```python
from build123d import *

# Parameters (mm, degrees)
F1_DEPTH = 63.5
F0_R     = 63.6308259599
F0_R_2   = 52.2581940634
F0_W     = 24.2178440094
F0_H     = 175.5797639489
F0_W_2   = 299.6964156628
F0_H_2   = 33.2996025681
F2_DEPTH = 6.35
F5_DEPTH = 25.4
F6_DEPTH = 19.05


# Not quite as in the source:
# - the program builds the solid bodies; features that only make, move or delete a surface that nothing else refers to are left out


with BuildPart() as f1:
    # F0 (on Front) → F1 (new body)
    with BuildSketch(Plane.XZ):
        Polygon((-969.1663980484, 198.6485360199), (-921.1349980484, 198.6485360199), (907.6650019516, 198.6485360199), (955.6964019516, 198.6485360199), (956.6172361374, 198.6485360199), (956.6172361374, 246.6799360199), (-969.1663980484, 246.6799360199), align=None)
        Polygon((-921.1349980484, -371.5092837811), (-921.1349980484, 198.6485360199), (-969.1663980484, 198.6485360199), (-969.1663980484, -410.9517233025), (-921.1349980484, -410.9517233025), (-921.1349980484, -410.9514639801), align=None)
        Polygon((-921.1349980484, -410.9517233025), (-969.1663980484, -410.9517233025), (-969.1663980484, -458.9831233025), (955.726981163, -458.9831233025), (955.726981163, -410.9517233025), (955.6964019516, -410.9517233025), (907.6650019516, -410.9517233025), align=None)
        Polygon((955.6964019516, 198.6485360199), (907.6650019516, 198.6485360199), (907.6650019516, -410.9514639801), (907.6650019516, -410.9517233025), (955.6964019516, -410.9517233025), align=None)
    extrude(amount=F1_DEPTH)

    # F0 (on Front) → F2 (join)
    with BuildSketch(Plane.XZ):
        Polygon((907.6650019516, 198.6485360199), (-921.1349980484, 198.6485360199), (-921.1349980484, -371.5092837811), (-921.1349980484, -410.9514639801), (-31.4717553556, -410.9514639801), (907.6650019516, -410.9514639801), align=None)
        Polygon((-789.5849161051, -398.2566583191), (-795.2640652657, -368.8750267029), (-420.4561412334, -296.4287400246), (-420.4561412334, -326.9080892764), align=None, mode=Mode.SUBTRACT)
        Polygon((210.169616585, -380.4944990589), (206.6856175661, -339.3833041191), (563.899576664, -309.1109395027), (566.059074651, -350.3343802749), align=None, mode=Mode.SUBTRACT)
        Polygon((235.5920225382, -246.5991973877), (81.9196328521, -266.643434763), (78.3429656397, -239.222336751), (239.8227507102, -218.1597428141), align=None, mode=Mode.SUBTRACT)
        with Locations((470.1542854309, -190.9026801586)):
            Circle(F0_R, mode=Mode.SUBTRACT)
        with Locations((836.3508582115, -221.3210761547)):
            Circle(F0_R_2, mode=Mode.SUBTRACT)
        with Locations((-737.8122806549, 54.1574768722)):
            Rectangle(F0_W, F0_H, mode=Mode.SUBTRACT)
        Polygon((-614.0667200089, 62.5602602959), (-606.2821745872, 91.4887040854), (-299.1916835308, 14.3223749474), (-307.1056894279, -17.1721380653), align=None, mode=Mode.SUBTRACT)
        Polygon((777.5867510857, 41.2790888272), (818.6616301537, 58.8090009987), (872.9156851768, -56.7944645882), (832.5127084301, -75.7560529142), align=None, mode=Mode.SUBTRACT)
        Polygon((-132.3649287224, 135.8928531408), (109.8140254617, 135.8928531408), (167.3315316439, 81.402592361), (-68.7929466367, 81.402592361), align=None, mode=Mode.SUBTRACT)
        with Locations((625.9579211473, 125.2975575626)):
            Rectangle(F0_W_2, F0_H_2, mode=Mode.SUBTRACT)
        Polygon((907.6650019516, -410.9517233025), (907.6650019516, -410.9514639801), (-31.4717553556, -410.9514639801), (-921.1349980484, -410.9514639801), (-921.1349980484, -410.9517233025), align=None)
    extrude(amount=F2_DEPTH)

    # F0 (on Front) → F5 (join)
    with BuildSketch(Plane.XZ):
        with Locations((625.9579211473, 125.2975575626)):
            Rectangle(F0_W_2, F0_H_2)
        Polygon((167.3315316439, 81.402592361), (109.8140254617, 135.8928531408), (-132.3649287224, 135.8928531408), (-68.7929466367, 81.402592361), align=None)
        Polygon((-299.1916835308, 14.3223749474), (-606.2821745872, 91.4887040854), (-614.0667200089, 62.5602602959), (-307.1056894279, -17.1721380653), align=None)
        Polygon((-420.4561412334, -296.4287400246), (-795.2640652657, -368.8750267029), (-789.5849161051, -398.2566583191), (-420.4561412334, -326.9080892764), align=None)
        Polygon((78.3429656397, -239.222336751), (81.9196328521, -266.643434763), (235.5920225382, -246.5991973877), (239.8227507102, -218.1597428141), align=None)
        Polygon((563.899576664, -309.1109395027), (206.6856175661, -339.3833041191), (210.169616585, -380.4944990589), (566.059074651, -350.3343802749), align=None)
        with Locations((-737.8122806549, 54.1574768722)):
            Rectangle(F0_W, F0_H)
        Polygon((872.9156851768, -56.7944645882), (818.6616301537, 58.8090009987), (777.5867510857, 41.2790888272), (832.5127084301, -75.7560529142), align=None)
    extrude(amount=F5_DEPTH)

    # F0 (on Front) → F6 (join)
    with BuildSketch(Plane.XZ):
        with Locations((470.1542854309, -190.9026801586)):
            Circle(F0_R)
    extrude(amount=F6_DEPTH)


solid = f1.part
```
Verification items for the finished model (mm, model axes). A direction names the side the tool comes from. Round coordinates to 2 decimals unless told otherwise and drop trailing zeros. Write each loop counter-clockwise with the first axis right and the second up, starting at its lowest first coordinate (ties: lowest second). Pieces come first, ordered by that corner, then holes. Notation, with made-up numbers: (-6.5, 33.5) -> (9.5, 33.5) arc R10 cw to (9.5, 40.5) -> close; hole circle Ø7 at (53.5, -9). An arc over 180 degrees is marked (long way). Write each question's results on one line, items separated by ' | '. Start each with the question number.
1. Material ranges on probe 1 along X at (y, z) = (-20, -121) (3 decimals); probe 2 along Z at (x, y) = (336, -30.5); probe 3 along Y at (x, z) = (76.5, 93.5), recorded low to high. Write a range as from..to.
2. Draft check along Z on faces 1 (the flat face through (7, -31, 246.68)), 2 (the flat face through (955.696, -31, -110)), 3 (the cylindrical face through (528.933, -12.611, -215.274)), 4 (the flat face through (-605.236, -15.742, -332.145)). Enter one of: +Z half, -Z half, draft (parallel to the pull), parting line (faces both ways), or undercut.
3. Cross-section at B-B (z = -100.5). Enter the section's corners in (x, y) (3 decimals).
4. Cross-section at D-D (x = -502). Enter the section's corners in (y, z).
5. Cross-section at C-C (x = 695). Enter the section's corners in (y, z), then the cut area to 3 significant figures.
6. Cross-section at A-A (y = -37). Enter the section's corners in (x, z) (3 decimals).
7. Set-up check for faces 5 (the flat face through (956.617, -31, 222)), 6 (the flat face through (384, -25.4, -344)): record each of +Z, -Z, +X, -X, +Y, -Y from which the full face is reachable in a straight line by a thin tool's end or side.
8. Depth check by flat-ended pin: P1, Ø21.5, axis at x = 415, z = -332.5, coming from the -Y side; P2, Ø1, axis at y = -50.5, z = -49.5, coming from the +X side; P3, Ø1.5, axis at x = -751.5, z = -290.5, coming from the -Y side; P4, Ø1.5, axis at x = -294, z = 152, coming from the +Y side. Enter the tip coordinate at first touch or a pass-through.
Solutions:
1) probe 1: x = -969.166..-921.135, 907.665..955.696 | probe 2: z = -458.98..-410.95, 198.65..246.68 | probe 3: y = -25.4..0
2) face 1: +Z half | face 2: draft | face 3: undercut | face 4: undercut
3) outline: (-969.166, -63.5) -> (-921.135, -63.5) -> (-921.135, -6.35) -> (907.665, -6.35) -> (907.665, -63.5) -> (955.696, -63.5) -> (955.696, 0) -> (-969.166, 0) -> close
4) outline: (-63.5, -458.98) -> (0, -458.98) -> (0, 246.68) -> (-63.5, 246.68) -> (-63.5, 198.65) -> (-6.35, 198.65) -> (-6.35, 65.28) -> (-25.4, 65.28) -> (-25.4, 33.45) -> (-6.35, 33.45) -> (-6.35, -312.19) -> (-25.4, -312.19) -> (-25.4, -342.67) -> (-6.35, -342.67) -> (-6.35, -410.95) -> (-63.5, -410.95) -> close
5) outline: (-63.5, -458.98) -> (0, -458.98) -> (0, 246.68) -> (-63.5, 246.68) -> (-63.5, 198.65) -> (-6.35, 198.65) -> (-6.35, 141.95) -> (-25.4, 141.95) -> (-25.4, 108.65) -> (-6.35, 108.65) -> (-6.35, -410.95) -> (-63.5, -410.95) -> close | area: 10,600 mm2
6) outline: (-969.166, -458.983) -> (955.727, -458.983) -> (955.727, -410.952) -> (955.696, -410.952) -> (955.696, 198.649) -> (956.617, 198.649) -> (956.617, 246.68) -> (-969.166, 246.68) -> close; hole (-921.135, -410.952) -> (907.665, -410.952) -> (907.665, 198.649) -> (-921.135, 198.649) -> close
7) face 5: +Z, -Z, +X, +Y, -Y | face 6: -Y
8) P1: stops at y = -25.4 | P2: stops at x = 955.7 | P3: stops at y = -6.35 | P4: stops at y = 0
